Part model, mm, in its own coordinate system. Give positions to 0.01 mm unless a question says otherwise; leave off trailing zeros. Order: outer loops, then holes, each group sorted by start corner. A loop starts at its lowest first (then second) coordinate and runs counter-clockwise, first axis right, second up.
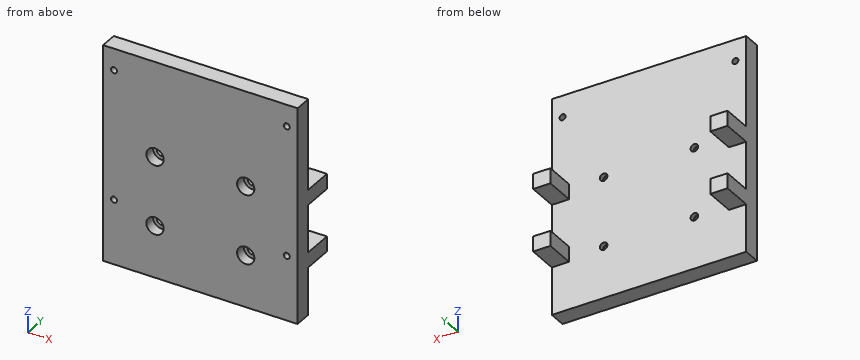
Solid Edge part; units mm, degrees
sketch "Sketch1" plane through (0, 0, 0) normal (0, -1, 0) x (1, 0, 0)
  line L0 (-45, -40) -> (45, -40)
  line L1 (45, -40) -> (45, 40)
  line L2 (45, 40) -> (-45, 40)
  line L3 (-45, 40) -> (-45, -40)
  dimension "D1" = 45
  dimension "D2" = 45
extrude "Protrusion1" add sketch "Sketch1" against normal blind 8
sketch "Sketch2" plane through (0, 0, 0) normal (0, -1, 0) x (1, 0, 0)
  circle A0 centre (-21, 16) radius 4
  circle A1 centre (-21, -16) radius 4
  circle A2 centre (21, -16) radius 4
  circle A3 centre (21, 16) radius 4
extrude "Extrusionsausschnitt_2" cut sketch "Sketch2" against normal blind 5
sketch "Sketch3" plane through (0, 0, 0) normal (0, -1, 0) x (1, 0, 0)
  circle A0 centre (-21, 16) radius 1.75
  circle A1 centre (-21, -16) radius 1.75
  circle A2 centre (21, -16) radius 1.75
  circle A3 centre (21, 16) radius 1.75
extrude "Cutout1" cut sketch "Sketch3" against normal through all
chamfer "Fase_1" [suppressed]
chamfer "Fase_2" [suppressed]
chamfer "Fase_4" distance 0.5 angle 60 4 edges at (-21, 5, 14.25) (-21, 5, -17.75) (21, 5, 14.25) (21, 5, -17.75) measured on face at (-23.5867, 5, 18.7467) measured on face at (-23.5867, 5, -13.2533) measured on face at (18.4133, 5, 18.7467) measured on face at (18.4133, 5, -13.2533)
sketch "Sketch4" plane through (0, 8, 0) normal (0, 1, 0) x (1, 0, 0)
  line L0 (-45, 11) -> (-37, 11)
  line L1 (-37, 11) -> (-37, 18)
  line L2 (-37, 18) -> (-45, 18)
  line L3 (-45, 18) -> (-45, 11)
  dimension "D1" = 45
  dimension "D2" = 45
extrude "Extrusionsausprägung_2" add sketch "Sketch4" along normal blind 14
mirror "Mirror1" about plane through (0, 0, 0) normal (0, 0, 1) of "Extrusionsausprägung_2"
mirror "Mirror2" about plane through (0, 0, 0) normal (1, 0, 0) of "Extrusionsausprägung_2", "Mirror1"
sketch "Sketch5" plane through (0, 0, 0) normal (0, -1, 0) x (-1, 0, 0)
  line L0 (-45, -40) -> (45, -40)
  line L1 (45, -40) -> (45, -60)
  line L2 (45, -60) -> (-45, -60)
  line L3 (-45, -60) -> (-45, -40)
  dimension "D1" = 45
extrude "Protrusion5" add sketch "Sketch5" against normal up to vertex (8 mm away)
sketch "Sketch6" plane through (0, 0, 0) normal (0, -1, 0) x (1, 0, 0)
  circle A0 centre (-40, -10) radius 1.4
  circle A1 centre (40, -10) radius 1.4
  circle A2 centre (40, 50) radius 1.4
  circle A3 centre (-40, 50) radius 1.4
  dimension "D1" = 40
  dimension "D2" = 40
extrude "Cutout2" cut sketch "Sketch6" against normal up to vertex (8 mm away)
properties material "Nylon, allgemein"
Item 1: Drop flat-ended pins along their axis: P1, Ø2, axis at x = -2, z = -25.5, coming from the +Y side; P2, Ø6, axis at y = 11.5, z = 39.5, coming from the +X side; P3, Ø2.5, axis at x = 19, z = 15, coming from the -Y side; P4, Ø2.5, axis at x = 43, y = 16, coming from the +Z side. Give the stop position or say it passes through.
Item 2: Band-saw the part on A-A on x = 21. List the corners of the cut face in (y, z), plus the area to 3 significant figures.
Item 3: Band-saw the part on D-D on z = 50. List the corners of the cut face in (x, y), plus the area to 3 significant figures.
Item 4: Band-saw the part on C-C on y = 20.5. List the corners of the cut face in (x, z), plus the area to 3 significant figures.
Item 5: Band-saw the part on B-B on z = 16. List the corners of the cut face in (x, y), plus the area to 3 significant figures.
Item 6: Drill centre lines: probe 1 along Z at (x, y) = (-21, 1.5); probe 2 along X at (y, z) = (2.5, -10); probe 3 along Z at (x, y) = (21, 6.9). Where is each one in solid material? Low to high.
Working result:
1. P1: stops at y = 8
1. P2: passes through
1. P3: stops at y = 5
1. P4: stops at z = 18
2. outline: (0, -40) - (8, -40) - (8, -17.75) - (5.87, -17.75) - (5, -18.25) - (5, -20) - (0, -20) - close; (0, -12) - (5, -12) - (5, -13.75) - (5.87, -14.25) - (8, -14.25) - (8, 14.25) - (5.87, 14.25) - (5, 13.75) - (5, 12) - (0, 12) - close; (0, 20) - (5, 20) - (5, 18.25) - (5.87, 17.75) - (8, 17.75) - (8, 60) - (0, 60) - close
2. area: 698 mm2
3. outline: (-45, 0) - (-41.4, 0) - (-41.4, 8) - (-45, 8) - close; (-38.6, 0) - (38.6, 0) - (38.6, 8) - (-38.6, 8) - close; (41.4, 0) - (45, 0) - (45, 8) - (41.4, 8) - close
3. area: 675 mm2
4. outline: (-45, -18) - (-37, -18) - (-37, -11) - (-45, -11) - close; (-45, 11) - (-37, 11) - (-37, 18) - (-45, 18) - close; (37, -18) - (45, -18) - (45, -11) - (37, -11) - close; (37, 11) - (45, 11) - (45, 18) - (37, 18) - close
4. area: 224 mm2
5. outline: (-45, 0) - (-25, 0) - (-25, 5) - (-23.25, 5) - (-22.75, 5.87) - (-22.75, 8) - (-37, 8) - (-37, 22) - (-45, 22) - close; (-19.25, 5.87) - (-18.75, 5) - (-17, 5) - (-17, 0) - (17, 0) - (17, 5) - (18.75, 5) - (19.25, 5.87) - (19.25, 8) - (-19.25, 8) - close; (22.75, 5.87) - (23.25, 5) - (25, 5) - (25, 0) - (45, 0) - (45, 22) - (37, 22) - (37, 8) - (22.75, 8) - close
5. area: 842 mm2
6. probe 1: z = -40 to -20, -12 to 12, 20 to 60
6. probe 2: x = -45 to -41.4, -38.6 to 38.6, 41.4 to 45
6. probe 3: z = -40 to -17.75, -14.25 to 14.25, 17.75 to 60
